```python
from build123d import *

# Parameters (mm, degrees)
F0_W     = 34
F0_H     = 7
F1_DEPTH = 2.4
F2_W     = 4.25
F2_H     = 16.6
F3_DEPTH = 7
F5_DEPTH = 10
F6_R     = 4


# Not quite as in the source:
# - a pattern or mirror of a feature is missing from the dataset's text; its kind, count and spacing are read off the source's solid


with BuildPart() as f1:
    # F0 (on Top) → F1 (new body)
    with BuildSketch(Plane.XY):
        Rectangle(F0_W, F0_H)
    extrude(amount=F1_DEPTH)

    # F2 (on face) → F3 (join)
    with BuildSketch(Plane(origin=(0, 3.5, 0), x_dir=(-1, 0, 0), z_dir=(0, 1, 0))):
        with Locations((14.875, -8.3)):
            Rectangle(F2_W, F2_H)
        with Locations((-14.875, -8.3)):
            Rectangle(F2_W, F2_H)
    extrude(amount=-F3_DEPTH)

    # F4 (on face) → F5 (cut)
    with BuildSketch(Plane(origin=(0, 3.5, 0), x_dir=(-1, 0, 0), z_dir=(0, 1, 0))):
        Polygon((12.75, -12.6), (12.75, -16.6), (13.95, -16.6), (13.95, -15), (15.15, -13.8), (15.15, -12.6), align=None)
    f5 = extrude(amount=-F5_DEPTH, mode=Mode.SUBTRACT)

    # F5_copies: F5 across plane
    add(f5.mirror(Plane(origin=(0, 0, 0), x_dir=(0, 0, 1), z_dir=(1, 0, 0))), mode=Mode.SUBTRACT)

    # F6
    f6_edges = [f1.edges().sort_by_distance(p)[0] for p in [
        (17, 0, 2.4),
        (-17, 0, 2.4),
    ]]
    fillet(f6_edges, radius=F6_R)


solid = f1.part
```
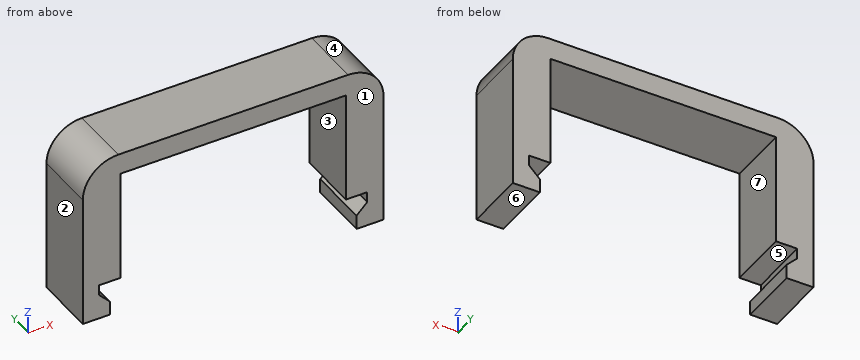
Verification items for the finished model (mm, model axes). Face numbers are marked on the shaded views. A direction names the side the tool comes from. Round coordinates to 2 decimals unless told otherwise and drop trailing zeros. Order: outer loops, then holes, each group sorted by start corner. A loop starts at its lowest first (then second) coordinate and runs counter-clockwise, first axis right, second up. Notation, with made-up numbers: (-14, 79.25) -> (32, 79.25) arc R21 cw to (32, 87.25) -> close; hole circle Ø1 at (-20, -0.75). An arc over 180 degrees is marked (long way). Put each result on its own line as item: value. Start each with the question number.
(1) Section check D-D (z = 1.25). Enter the section's corners in (x, y), then the cut area to 3 significant figures.
(2) Material ranges on line 1 along X through (y, z) = (1.75, -9.5); line 2 along X through (y, z) = (2.5, -16); line 3 along Z through (x, y) = (-3, 1.25), recorded low to high.
(3) Depth check by flat-ended pin: pin 1 Ø8 at (x, z) = (11, -9) entering from +Y; pin 2 Ø2 at (x, y) = (2, 0.5) entering from -Z; pin 3 Ø2 at (x, z) = (10, -13) entering from +Y. Enter the tip coordinate at first touch or a pass-through.
(4) Section check C-C (x = -5.5). Enter the section's corners in (y, z).
(5) Tool access check on the marked faces 5, 6 and 7. Record the directions out of +Z, -Z, +X, -X, +Y, -Y that give a thin tool (end or side, any length) a straight path to the whole face; none if there is none.
(6) Section check A-A (z = -11.75). Enter the section's corners in (x, y), then the cut area to 3 significant figures.
(7) Section check B-B (y = 1.5). Enter the section's corners in (x, z), then the cut area to 3 significant figures.
(8) Draft check along X on the marked faces 1, 2, 3 and 4. Enter one of: +X half, -X half, draft (parallel to the pull), parting line (faces both ways), or undercut.
Completed:
1. outline: (-15.81, -3.5) -> (15.81, -3.5) -> (15.81, 3.5) -> (-15.81, 3.5) -> close
1. area: 221 mm2
2. line 1: x = -17 to -12.75, 12.75 to 17
2. line 2: x = -17 to -13.95, 13.95 to 17
2. line 3: z = 0 to 2.4
3. pin 1: stops at y = 3.5
3. pin 2: stops at z = 0
3. pin 3: passes through
4. outline: (-3.5, 0) -> (3.5, 0) -> (3.5, 2.4) -> (-3.5, 2.4) -> close
5. face 5: +Y, -Y
5. face 6: -Z, +X, -X, +Y, -Y
5. face 7: -Z, +Y, -Y
6. outline: (-17, -3.5) -> (-12.75, -3.5) -> (-12.75, 3.5) -> (-17, 3.5) -> close; (12.75, -3.5) -> (17, -3.5) -> (17, 3.5) -> (12.75, 3.5) -> close
6. area: 59.5 mm2
7. outline: (-17, -16.6) -> (-13.95, -16.6) -> (-13.95, -15) -> (-15.15, -13.8) -> (-15.15, -12.6) -> (-12.75, -12.6) -> (-12.75, 0) -> (12.75, 0) -> (12.75, -12.6) -> (15.15, -12.6) -> (15.15, -13.8) -> (13.95, -15) -> (13.95, -16.6) -> (17, -16.6) -> (17, -1.6) arc R4 ccw to (13, 2.4) -> (-13, 2.4) arc R4 ccw to (-17, -1.6) -> close
7. area: 202 mm2
8. face 1: draft
8. face 2: -X half
8. face 3: undercut
8. face 4: +X half
